```python
from build123d import *

# Parameters (mm, degrees)
SKETCH1_R                = 17.5
SKETCH1_R_2              = 10
SKETCH1_W                = 4.9
SKETCH1_H                = 1.992179872
SKETCH1_W_2              = 1.992179872
SKETCH1_H_2              = 4.9
BOSS_EXTRUDE1_DEPTH      = 0.8
BOSS_EXTRUDE1_DEPTH_BACK = 0.8


with BuildPart() as part:
    # Sketch1 → Boss-Extrude1 (new body, two sides)
    with BuildSketch(Plane(origin=(0, 0, 0), x_dir=(0, 0, -1), z_dir=(1, 0, 0))) as boss_extrude1_sk:
        Circle(SKETCH1_R)
        Circle(SKETCH1_R_2, mode=Mode.SUBTRACT)
        with Locations((13.725, 0)):
            Rectangle(SKETCH1_W, SKETCH1_H, mode=Mode.SUBTRACT)
        Polygon((10.633006645, 3.880333728), (11.148620737, 1.956035739), (15.881657286, 3.22424906), (15.366043194, 5.148547049), align=None, mode=Mode.SUBTRACT)
        Polygon((10.633006645, -3.880333728), (15.366043194, -5.148547049), (15.881657286, -3.22424906), (11.148620737, -1.956035739), align=None, mode=Mode.SUBTRACT)
        Polygon((9.26639146, 6.500139189), (10.262481396, 4.774860811), (14.506005874, 7.224860811), (13.509915938, 8.950139189), align=None, mode=Mode.SUBTRACT)
        Polygon((9.26639146, -6.500139189), (13.509915938, -8.950139189), (14.506005874, -7.224860811), (10.262481396, -4.774860811), align=None, mode=Mode.SUBTRACT)
        Polygon((7.26828701, 8.676970906), (8.676970906, 7.26828701), (12.141794134, 10.733110237), (10.733110237, 12.141794134), align=None, mode=Mode.SUBTRACT)
        Polygon((7.26828701, -8.676970906), (10.733110237, -12.141794134), (12.141794134, -10.733110237), (8.676970906, -7.26828701), align=None, mode=Mode.SUBTRACT)
        Polygon((4.774860811, 10.262481396), (6.500139189, 9.26639146), (8.950139189, 13.509915938), (7.224860811, 14.506005874), align=None, mode=Mode.SUBTRACT)
        Polygon((4.774860811, -10.262481396), (7.224860811, -14.506005874), (8.950139189, -13.509915938), (6.500139189, -9.26639146), align=None, mode=Mode.SUBTRACT)
        Polygon((1.956035739, 11.148620737), (3.880333728, 10.633006645), (5.148547049, 15.366043194), (3.22424906, 15.881657286), align=None, mode=Mode.SUBTRACT)
        Polygon((1.956035739, -11.148620737), (3.22424906, -15.881657286), (5.148547049, -15.366043194), (3.880333728, -10.633006645), align=None, mode=Mode.SUBTRACT)
        with Locations((0, 13.725)):
            Rectangle(SKETCH1_W_2, SKETCH1_H_2, mode=Mode.SUBTRACT)
        with Locations((0, -13.725)):
            Rectangle(SKETCH1_W_2, SKETCH1_H_2, mode=Mode.SUBTRACT)
        Polygon((-5.148547049, 15.366043194), (-3.880333728, 10.633006645), (-1.956035739, 11.148620737), (-3.22424906, 15.881657286), align=None, mode=Mode.SUBTRACT)
        Polygon((-5.148547049, -15.366043194), (-3.22424906, -15.881657286), (-1.956035739, -11.148620737), (-3.880333728, -10.633006645), align=None, mode=Mode.SUBTRACT)
        Polygon((-8.950139189, 13.509915938), (-6.500139189, 9.26639146), (-4.774860811, 10.262481396), (-7.224860811, 14.506005874), align=None, mode=Mode.SUBTRACT)
        Polygon((-8.950139189, -13.509915938), (-7.224860811, -14.506005874), (-4.774860811, -10.262481396), (-6.500139189, -9.26639146), align=None, mode=Mode.SUBTRACT)
        Polygon((-12.141794134, 10.733110237), (-8.676970906, 7.26828701), (-7.26828701, 8.676970906), (-10.733110237, 12.141794134), align=None, mode=Mode.SUBTRACT)
        Polygon((-12.141794134, -10.733110237), (-10.733110237, -12.141794134), (-7.26828701, -8.676970906), (-8.676970906, -7.26828701), align=None, mode=Mode.SUBTRACT)
        Polygon((-14.506005874, 7.224860811), (-10.262481396, 4.774860811), (-9.26639146, 6.500139189), (-13.509915938, 8.950139189), align=None, mode=Mode.SUBTRACT)
        Polygon((-14.506005874, -7.224860811), (-13.509915938, -8.950139189), (-9.26639146, -6.500139189), (-10.262481396, -4.774860811), align=None, mode=Mode.SUBTRACT)
        Polygon((-15.881657286, 3.22424906), (-11.148620737, 1.956035739), (-10.633006645, 3.880333728), (-15.366043194, 5.148547049), align=None, mode=Mode.SUBTRACT)
        Polygon((-15.881657286, -3.22424906), (-15.366043194, -5.148547049), (-10.633006645, -3.880333728), (-11.148620737, -1.956035739), align=None, mode=Mode.SUBTRACT)
        with Locations((-13.725, 0)):
            Rectangle(SKETCH1_W, SKETCH1_H, mode=Mode.SUBTRACT)
    extrude(amount=BOSS_EXTRUDE1_DEPTH)
    extrude(boss_extrude1_sk.sketch, amount=-BOSS_EXTRUDE1_DEPTH_BACK)


solid = part.part
```
Can you work these out from the model? Positions are in its coordinate system, mm. Give positions to 0.01 mm unless a question says otherwise; leave off trailing zeros. Order: outer loops, then holes, each group sorted by start corner. A loop starts at its lowest first (then second) coordinate and runs counter-clockwise, first axis right, second up. Notation, with made-up numbers: M 64,55.25 L 95,55.25 A19 cw 95,92.25 Z; hole C 67.25,30 d1. An arc over 180 degrees is marked long. One line per item, written item: value.
1) I want a section at C-C, the plane z = 8. List the corners of the cut face in (x, y) for me, plus the area to 3 significant figures.
Answer sheet:
outline: M -0.8,-15.56 L 0.8,-15.56 L 0.8,-14.06 L -0.8,-14.06 Z; M -0.8,-11.86 L 0.8,-11.86 L 0.8,-9.41 L -0.8,-9.41 Z; M -0.8,-7.95 L 0.8,-7.95 L 0.8,-6 L -0.8,-6 Z; M -0.8,6 L 0.8,6 L 0.8,7.95 L -0.8,7.95 Z; M -0.8,9.41 L 0.8,9.41 L 0.8,11.86 L -0.8,11.86 Z; M -0.8,14.06 L 0.8,14.06 L 0.8,15.56 L -0.8,15.56 Z
area: 18.9 mm^2
2) I want a section at A-A, the plane z = 0. List the corners of the cut face in (x, y) for me (3 decimals), plus the area to 3 significant figures.
Answer sheet:
outline: M -0.8,-17.5 L 0.8,-17.5 L 0.8,-16.175 L -0.8,-16.175 Z; M -0.8,-11.275 L 0.8,-11.275 L 0.8,-10 L -0.8,-10 Z; M -0.8,10 L 0.8,10 L 0.8,11.275 L -0.8,11.275 Z; M -0.8,16.175 L 0.8,16.175 L 0.8,17.5 L -0.8,17.5 Z
area: 8.32 mm^2
3) Please list where these lines run through material, in increasing order: line 1 along Y through (x, z) = (-0.15, 0) (3 decimals); line 2 along Z through (x, y) = (-0.15, -6).
Answer sheet:
line 1: y = -17.5 to -16.175, -11.275 to -10, 10 to 11.275, 16.175 to 17.5
line 2: z = -16.44 to -12.38, -9.56 to -8, 8 to 9.56, 12.38 to 16.44
4) For P1, Ø0.5, axis at x = 0, y = -13, coming from the +Z side; P2, Ø0.8, axis at x = 0, z = -14, coming from the +Y side; P3, Ø0.8, axis at x = -0.5, z = 13, coming from the +Y side, each with a flat end and sliding along its axis, tell me the tip position at first contact or that it passes through.
Answer sheet:
P1: stops at z = 11.99
P2: stops at y = 11.01
P3: stops at y = 12.14
5) I want a section at D-D, the plane x = -0.25. Count the separate pieces of the cut face and the enclosed holes in it, plus the area to 3 significant figures.
Answer sheet:
separate pieces: 1
enclosed holes: 25
area: 414 mm^2
